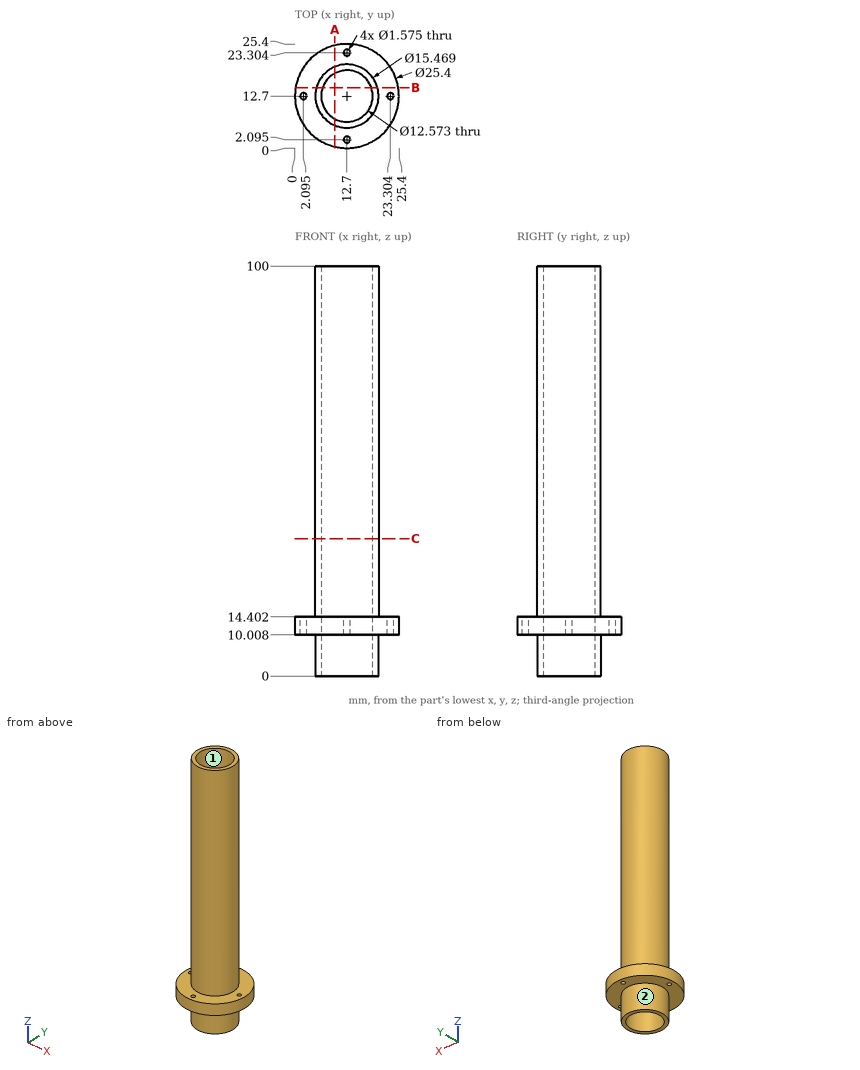
Job drawing, mm, ordinate dimensions from the low corner. One solid piece. Round coordinates to 2 decimals unless told otherwise and drop trailing zeros. Loops run counter-clockwise (first coordinate to the right, second up) from the corner with the lowest first, then second, coordinate; pieces in that order, holes last. Notation, with made-up numbers: (26, 33.5) -> (32, 33.5) arc R29 ccw to (32, 72.5) -> close; hole circle Ø6 at (-30, 30). An arc over 180 degrees is marked (long way). Use CSV: the item, a comma, the result in double quotes. Start each with the question number.
Q1. Saw through at A-A on x = 9.75. Give the cut face in (y, z).
Q2. Saw through at C-C on z = 33.5. Give the cut face in (x, y) (1 decimal).
Q3. Saw through at B-B on y = 14.75. Give the cut face in (x, z).
Q4. Flat gauge pins, fed straight in: pin 1 Ø5 at (y, z) = (22, 50.5) entering from -X (1 decimal); pin 2 Ø2 at (y, z) = (19, 48) entering from -X; pin 3 Ø1.8 at (x, y) = (23.3, 12.7) entering from +Z. Where does each tip first touch, or does it go through?
Q5. Mould opens along X. For the marked faces 1 and 2 say: +X half, -X half, draft (parallel to the pull), parting line (faces both ways), or undercut.
Q6. Drill centre lines: L1, parallel to Y at x = 12.7, z = 13.1; L2, parallel to Z at x = 4.75, y = 3.5; L3, parallel to Y at x = 17, z = 15.5 (1 decimal). Where is each one in solid material? Low to high.
Solutions:
1,outline,"(0.35, 10.01) -> (5.55, 10.01) -> (5.55, 0) -> (7.15, 0) -> (7.15, 100) -> (5.55, 100) -> (5.55, 14.4) -> (0.35, 14.4) -> close; (18.25, 0) -> (19.85, 0) -> (19.85, 10.01) -> (25.05, 10.01) -> (25.05, 14.4) -> (19.85, 14.4) -> (19.85, 100) -> (18.25, 100) -> close"
2,outline,"circle Ø15.5 at (12.7, 12.7); hole circle Ø12.6 at (12.7, 12.7)"
3,outline,"(0.17, 10.01) -> (5.24, 10.01) -> (5.24, 0) -> (6.76, 0) -> (6.76, 100) -> (5.24, 100) -> (5.24, 14.4) -> (0.17, 14.4) -> close; (18.64, 0) -> (20.16, 0) -> (20.16, 10.01) -> (25.23, 10.01) -> (25.23, 14.4) -> (20.16, 14.4) -> (20.16, 100) -> (18.64, 100) -> close"
4,pin 1,"stops at x = 9"
4,pin 2,"stops at x = 7.07"
4,pin 3,"stops at z = 14.4"
5,face 1,"undercut"
5,face 2,"parting line"
6,L1,"y = 0 to 1.31, 2.88 to 6.41, 18.99 to 22.52, 24.09 to 25.4"
6,L2,"z = 10.01 to 14.4"
6,L3,"y = 6.3 to 8.1, 17.3 to 19.1"
